Source: three-view drawing plus pictorial views. Frame: mm from the lowest corner of the part. A direction names the side the tool comes from. Coordinates: 2 decimals unless noted, no trailing zeros. Write each loop counter-clockwise with the first axis right and the second up, starting at its lowest first coordinate (ties: lowest second). Pieces come first, ordered by that corner, then holes. Notation, with made-up numbers: M 39,30 L 59,30 A9 cw 59,41 Z; hole C -39.5,55 d8. An arc over 180 degrees is marked long. Write item = value, one per line. Start each with the question number.
Item 1: Section A-A on z = 25. Output: boundary loops of the cut face in (x, y).
Item 2: First-contact query: pin 1 Ø6 at (x, y) = (42.5, 7.5) entering from +Z (1 decimal); pin 2 Ø1 at (y, z) = (11, 33) entering from +X; pin 3 Ø19 at (x, z) = (30, 30) entering from -Y. Flat tips, straight axial feed; report the tip coordinate or a pass-through.
Item 3: Section C-C on z = 36.5. Output: boundary loops of the cut face in (x, y) (1 decimal), plus the area to 3 significant figures.
Item 4: Reachability of the marked faces 1 and 2 from +Z, -Z, +X, -X, +Y, -Y: full face, straight path, thin tool, end or side. Return the list, or none.
Item 5: Section D-D on y = 6.75. Output: boundary loops of the cut face in (x, z) (1 decimal), plus the area to 3 significant figures.
Item 6: Section B-B on x = 25. Output: boundary loops of the cut face in (y, z).
Item 7: Pull-direction query (X, two-part tool) for the marked faces 3, 4, 5 and 6; classes: +X half, -X half, draft (parallel to the pull), parting line (faces both ways), or undercut.
Item 8: Ray query, L1, parallel to Z at x = 24, y = 7.75 (1 decimal); L2, parallel to X at y = 12.05, z = 25; L3, parallel to X at y = 2.5, z = 46 (1 decimal). Return the intervals inside material, ascending. Write a range as [from, to].
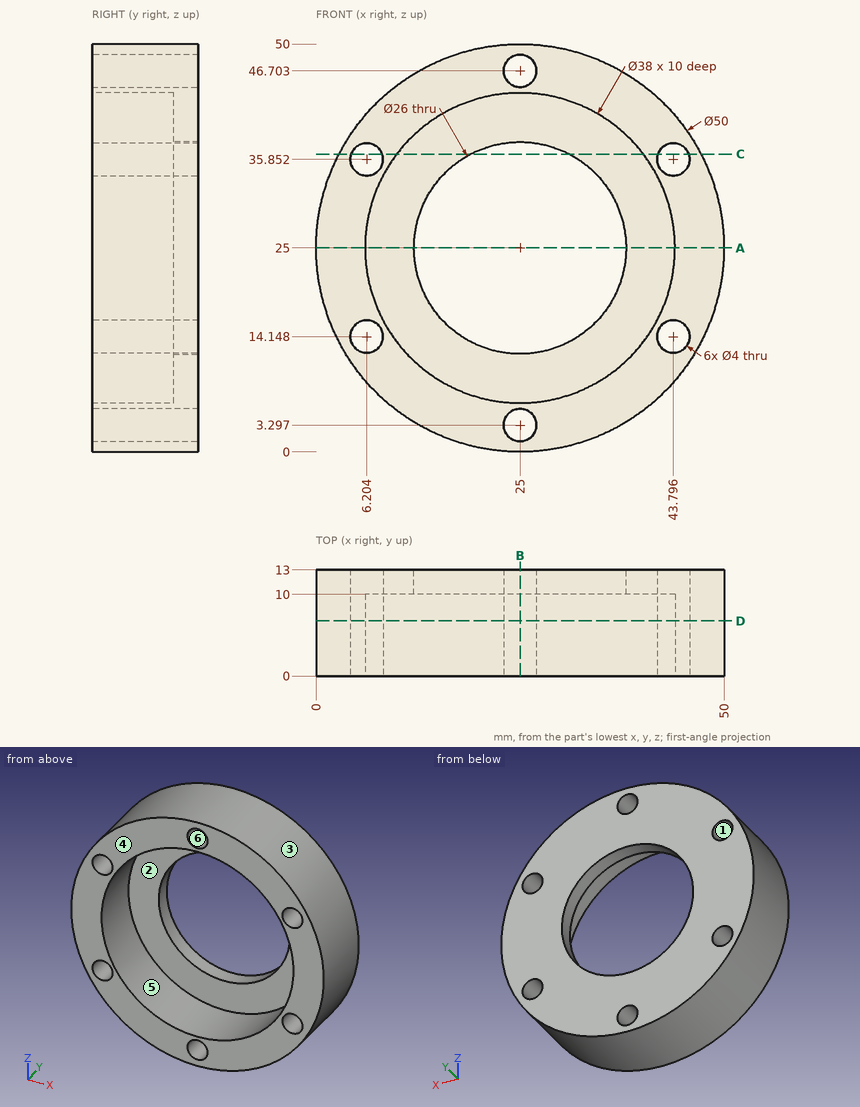
Responses:
q1.outline = M 0,0 L 6,0 L 6,10 L 12,10 L 12,13 L 0,13 Z; M 38,10 L 44,10 L 44,0 L 50,0 L 50,13 L 38,13 Z
q2.pin_1 = 45.4
q2.pin_2 = 48.85
q2.pin_3 = 10
q3.outline = M 2.8,0 L 4.3,0 L 4.3,13 L 2.8,13 Z; M 8.1,0 L 9.9,0 L 9.9,10 L 18.9,10 L 18.9,13 L 8.1,13 Z; M 31.1,10 L 40.1,10 L 40.1,0 L 41.9,0 L 41.9,13 L 31.1,13 Z; M 45.7,0 L 47.2,0 L 47.2,13 L 45.7,13 Z
q3.area = 140 mm²
q4.face_1 = +Y, -Y
q4.face_2 = -Y
q5.outline = C 25,25 d50; hole C 6.2,14.1 d4; hole C 6.2,35.9 d4; hole C 25,25 d38; hole C 25,3.3 d4; hole C 25,46.7 d4; hole C 43.8,14.1 d4; hole C 43.8,35.9 d4
q5.area = 754 mm²
q6.outline = M 0,0 L 13,0 L 13,1.3 L 0,1.3 Z; M 0,5.3 L 13,5.3 L 13,12 L 10,12 L 10,6 L 0,6 Z; M 0,44 L 10,44 L 10,38 L 13,38 L 13,44.7 L 0,44.7 Z; M 0,48.7 L 13,48.7 L 13,50 L 0,50 Z
q7.face_3 = parting line
q7.face_4 = draft
q7.face_5 = undercut
q7.face_6 = undercut
q8.L1 = [0, 1.6], [5, 6], [44, 45], [48.4, 50]
q8.L2 = [0, 12], [38, 50]
q8.L3 = [11.4, 23.1], [26.9, 38.6]
